from build123d import *

# Parameters (mm, degrees)
SKETCH_R           = 200
SKETCH_R_2         = 100
SKETCH_R_3         = 5
PAD_DEPTH          = 3
SKETCH001_W        = 3
SKETCH001_H        = 68
PAD001_DEPTH       = 84
SKETCH002_R        = 200
SKETCH002_R_2      = 127
SKETCH002_R_3      = 5
PAD002_DEPTH       = 3
POLARPATTERN_COUNT = 8
SKETCH003_W        = 20
SKETCH003_H        = 20
PAD003_DEPTH       = 10


with BuildPart() as part:
    # Sketch → Pad (new body)
    with BuildSketch(Plane.XY):
        Circle(SKETCH_R)
        Circle(SKETCH_R_2, mode=Mode.SUBTRACT)
        with Locations((-117.332701, 48.600796)):
            Circle(SKETCH_R_3, mode=Mode.SUBTRACT)
        with Locations((-48.600796, 117.332701)):
            Circle(SKETCH_R_3, mode=Mode.SUBTRACT)
        with Locations((48.600796, 117.332701)):
            Circle(SKETCH_R_3, mode=Mode.SUBTRACT)
        with Locations((117.332701, 48.600796)):
            Circle(SKETCH_R_3, mode=Mode.SUBTRACT)
        with Locations((117.332701, -48.600796)):
            Circle(SKETCH_R_3, mode=Mode.SUBTRACT)
        with Locations((48.600796, -117.332701)):
            Circle(SKETCH_R_3, mode=Mode.SUBTRACT)
        with Locations((-48.600796, -117.332701)):
            Circle(SKETCH_R_3, mode=Mode.SUBTRACT)
        with Locations((-117.332701, -48.600796)):
            Circle(SKETCH_R_3, mode=Mode.SUBTRACT)
    extrude(amount=PAD_DEPTH)

    # Sketch001 → Pad001 (join)
    with BuildSketch(Plane.XY):
        with Locations((-152, 0)):
            Rectangle(SKETCH001_W, SKETCH001_H)
    pad001 = extrude(amount=PAD001_DEPTH)

    # Sketch002 (on DatumPlane) → Pad002 (join)
    with BuildSketch(Plane.XY.offset(81)):
        Circle(SKETCH002_R)
        Circle(SKETCH002_R_2, mode=Mode.SUBTRACT)
        with Locations((-150, 90)):
            Circle(SKETCH002_R_3, mode=Mode.SUBTRACT)
        with Locations((-150, -90)):
            Circle(SKETCH002_R_3, mode=Mode.SUBTRACT)
        with Locations((150, 90)):
            Circle(SKETCH002_R_3, mode=Mode.SUBTRACT)
        with Locations((150, -90)):
            Circle(SKETCH002_R_3, mode=Mode.SUBTRACT)
    extrude(amount=PAD002_DEPTH)

    # PolarPattern: Pad001 ×8 about axis
    polarpattern_axis = Axis((0, 0, 0), (0, 0, 1))
    for i in range(1, POLARPATTERN_COUNT):
        add(pad001.rotate(polarpattern_axis, i * 360 / POLARPATTERN_COUNT))

    # Sketch003 (on DatumPlane) → Pad003 (join)
    with BuildSketch(Plane.XY.offset(81)):
        with Locations((170, 10)):
            Rectangle(SKETCH003_W, SKETCH003_H)
        with Locations((-10, 170)):
            Rectangle(SKETCH003_W, SKETCH003_H)
        with Locations((-170, -10)):
            Rectangle(SKETCH003_W, SKETCH003_H)
        with Locations((10, -170)):
            Rectangle(SKETCH003_W, SKETCH003_H)
    extrude(amount=PAD003_DEPTH)


solid = part.part
The listing builds one solid part. Answer for the finished solid, in the listing's coordinates (mm). A direction names the side the tool comes from. Coordinates: 2 decimals unless noted, no trailing zeros. Loops run counter-clockwise (first coordinate to the right, second up) from the corner with the lowest first, then second, coordinate; pieces in that order, holes last.
1) Find section D-D on y = -64.5. Write down the section's boundary in (x, z).
2) Find the intervals of material crossed by L1, parallel to Z at x = 133, y = 9; L2, parallel to Y at x = -4, z = 8.5; L3, parallel to Y at x = 0, z = 81.65, in increasing order.
3) Find section C-C on x = -5. Write down the section's boundary in (y, z), then the cut area to 3 significant figures.
4) Determine the mould class of faces 4 (the face through (-170, -10, 91)), 5 (the face through (0, 153.5, 41)), 6 (the face through (-117.98, 53.56, 1.48)) for opening direction Z: pulls with the +Z half, pulls with the -Z half, needs draft (parallel to the pull), parting line crosses it, or undercut.
5) A tool of negligible diameter and unlimited length cuts with its end or side. For faces 1 (the face through (-122.328, -48.381, 1.479)), 2 (the face through (108.2, 108.88, 41.45)), 3 (the face through (-106.76, 106.08, 41.45)), from which of +Z, -Z, +X, -X, +Y, -Y can it reach the whole face along a straight path? Write none if from no direction.
6) Find section A-A on z = 23. Give the number of separate pieces and of enclosed holes in the cut face, then the cut area to 3 significant figures.
7) Flat-ended cylindrical pins translate along their axes: pin 1 Ø4 at (y, z) = (-99, 28) entering from +X; pin 2 Ø20.5 at (y, z) = (-13, 33.5) entering from +X; pin 3 Ø11.5 at (x, y) = (150, -90) entering from -Z; pin 4 Ø10 at (y, z) = (22, 80.5) entering from +X. Find the tip coordinate at first contact, or state that the pin passes through.
Values:
1. outline: (-189.31, 0) - (-76.42, 0) - (-76.42, 3) - (-189.31, 3) - close; (-189.31, 81) - (-109.4, 81) - (-109.4, 84) - (-189.31, 84) - close; (76.42, 0) - (189.31, 0) - (189.31, 3) - (76.42, 3) - close; (109.4, 81) - (189.31, 81) - (189.31, 84) - (109.4, 84) - close
2. L1: z = 0 to 3, 81 to 84
2. L2: y = -153.5 to -150.5, 150.5 to 153.5
2. L3: y = -200 to -127, 127 to 200
3. outline: (-199.94, 0) - (-99.87, 0) - (-99.87, 3) - (-150.5, 3) - (-150.5, 81) - (-126.9, 81) - (-126.9, 84) - (-199.94, 84) - (-199.94, 81) - (-153.5, 81) - (-153.5, 3) - (-199.94, 3) - close; (99.87, 0) - (199.94, 0) - (199.94, 3) - (153.5, 3) - (153.5, 81) - (199.94, 81) - (199.94, 84) - (180, 84) - (180, 91) - (160, 91) - (160, 84) - (126.9, 84) - (126.9, 81) - (150.5, 81) - (150.5, 3) - (99.87, 3) - close
3. area: 1,650 mm2
4. face 4: pulls with the +Z half
4. face 5: undercut
4. face 6: needs draft
5. face 1: -Z
5. face 2: +X, +Y
5. face 3: none
6. separate pieces: 8
6. enclosed holes: 0
6. area: 1,630 mm2
7. pin 1: stops at x = 120.08
7. pin 2: stops at x = 153.5
7. pin 3: stops at z = 0
7. pin 4: stops at x = 199.27
